Input: part model. Units: mm. Frame: model coordinates. Face numbers are marked on the shaded views. Give positions to 0.01 mm unless a question says otherwise; leave off trailing zeros. Order: outer loops, then holes, each group sorted by start corner. A loop starts at its lowest first (then second) coordinate and runs counter-clockwise, first axis right, second up.
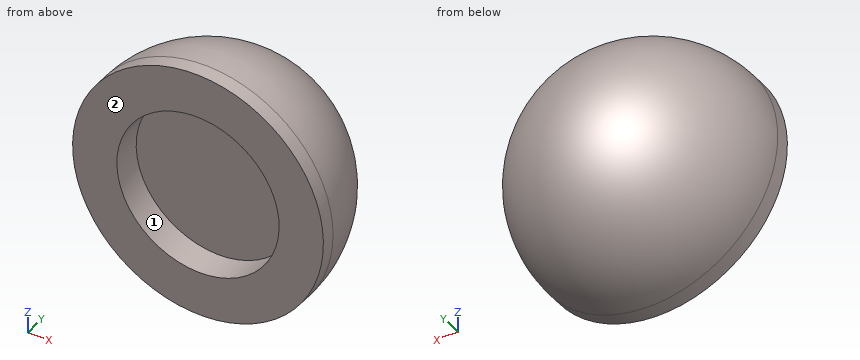
```python
from build123d import *

# Parameters (mm, degrees)
SKETCH1_R           = 17
BOSS_EXTRUDE1_DEPTH = 2
REVOLVE1_ANGLE      = 180
SKETCH3_R           = 11
CUT_EXTRUDE1_DEPTH  = 4


with BuildPart() as part:
    # Sketch1 → Boss-Extrude1 (new body)
    with BuildSketch(Plane(origin=(0, 0, 0), x_dir=(1, 0, 0), z_dir=(0, 1, 0))):
        with Locations(Location((0, 0, 0), (0, 0, 270))):
            Circle(SKETCH1_R)
    extrude(amount=BOSS_EXTRUDE1_DEPTH)

    # Sketch2 → Revolve1 (revolve)
    with BuildSketch(Plane(origin=(0, 2, 0), x_dir=(1, 0, 0), z_dir=(0, 1, 0))):
        with BuildLine():
            Line((-17, 0), (17, 0))
            ThreePointArc((17, 0), (0, 17), (-17, 0))
        make_face()
    revolve(axis=Axis((-17, 2, 0), (1, 0, 0)), revolution_arc=REVOLVE1_ANGLE)

    # Sketch3 → Cut-Extrude1 (cut)
    with BuildSketch(Plane.XZ):
        with Locations(Location((0, 0, 0), (0, 0, 270))):
            Circle(SKETCH3_R)
    extrude(amount=-CUT_EXTRUDE1_DEPTH, mode=Mode.SUBTRACT)


solid = part.part
```
1) Cut plane C-C (y = 3.5). Return the cut outline in (x, z).
2) Pull-direction query (X, two-part tool) for the marked faces 1 and 2; classes: pulls with the +X half, pulls with the -X half, needs draft (parallel to the pull), parting line crosses it, or undercut.
3) Line query: probe 1 along X at (y, z) = (2.1, 0); probe 2 along Z at (x, y) = (-0.5, 13); probe 3 along Y at (x, z) = (-9, -9.5). Output: solid intervals per line, ascending.
4) Cut plane A-A (x = 0). Return the cut outline in (y, z), then the cut area to 3 significant figures.
5) Cut plane D-D (y = 17.5). Return the cut outline in (x, z), then the cut area to 3 significant figures.
6) First-contact query: P1, Ø13, axis at x = 0, z = 0, coming from the -Y side; P2, Ø1, axis at y = 10.5, z = 4.5, coming from the -X side; P3, Ø6, axis at y = 9.5, z = 1.5, coming from the -X side. Flat tips, straight axial feed; report the tip coordinate or a pass-through.
7) Cut plane B-B (z = 0). Return the cut outline in (x, y), then the cut area to 3 significant figures.
Geometry says:
1. outline: circle Ø33.87 at (0, 0); hole circle Ø22 at (0, 0)
2. face 1: undercut
2. face 2: needs draft
3. probe 1: x = -17 to -11, 11 to 17
3. probe 2: z = -12.95 to 12.95
3. probe 3: y = 0 to 12.85
4. outline: (0, -17) - (2, -17) arc R17 ccw to (2, 17) - (0, 17) - (0, 11) - (4, 11) - (4, -11) - (0, -11) - close
4. area: 434 mm2
5. outline: circle Ø13.96 at (0, 0)
5. area: 153 mm2
6. P1: stops at y = 4
6. P2: stops at x = -14.35
6. P3: stops at x = -16.35
7. outline: (-17, 0) - (-11, 0) - (-11, 4) - (11, 4) - (11, 0) - (17, 0) - (17, 2) arc R17 ccw to (-17, 2) - close
7. area: 434 mm2
